Read the model definition and answer for the solid it produces. Units are mm, in the model's axes. A direction names the side the tool comes from. Coordinates: 2 decimals unless noted, no trailing zeros. Write each loop counter-clockwise with the first axis right and the second up, starting at its lowest first coordinate (ties: lowest second). Pieces come first, ordered by that corner, then holes.
(1) Which of the six approach directions +Z, -Z, +X, -X, +Y, -Y give full straight-line access (tool end or side, diameter ignored) to faces 5 (the flat face through (0, 5, 4)), 6 (the flat face through (-0.11, 8.09, -63.03)), 7 (the flat face through (-7.5, 3, -42)), 8 (the flat face through (42, 3, 7.5))?
(2) Given pin 1 (5 mm diameter, centred on x = 34.5, y = 6.5, fed in from -Z); pin 2 (8 mm diameter, centred on x = 3.5, z = -29, fed in from -Y), each flat-ended and moving along its own axis, determine where each tip first touches the part or whether it passes through.
(3) Determine the mould class of faces 1 (the cylindrical face through (-10.568, 2.465, 10.645)), 2 (the flat face through (42, 3, -7.5)), 3 (the flat face through (-7.5, 3, 42)), 4 (the cylindrical face through (63.49, 5.68, -0.09)) for opening direction Z: pulls with the +Z half, pulls with the -Z half, needs draft (parallel to the pull), parting line crosses it, or undercut.
(4) The part is cut by section C-C, the plane z = -49.5. Determine the outline of the cut face in (x, y).
(5) Straight lines are drawn through the part: line 1 along Y through (x, z) = (-7, -33); line 2 along X through (y, z) = (2, -23). For each, find the intervals that lie inside material, in ascending order.
(6) The part is cut by section A-A, the plane z = 0. Determine the outline of the cut face in (x, y).
(7) The part is cut by section B-B, the plane x = 0. Determine the outline of the cut face in (y, z).
(8) The part is cut by section D-D, the plane x = -31.5. Determine the outline of the cut face in (y, z), and give its area (3 significant figures).
```python
from build123d import *

# Parameters (mm, degrees)
EXTRUDE_1_DEPTH             = 5
EXTRUDE_6_DEPTH             = 15
EXTRUDE_7_DEPTH             = 15
EXTRUDE_8_DEPTH             = 15
EXTRUDE_9_DEPTH             = 15
HOLE_WIZARD_M61_D           = 5
HOLE_WIZARD_M51_D           = 4.2
HOLE_WIZARD_M51_ON_FACE_2_D = 4.2
HOLE_WIZARD_M51_ON_FACE_3_D = 4.2
HOLE_WIZARD_M51_ON_FACE_4_D = 4.2


with BuildPart() as part:
    # Эскиз1 → Бобышка-Вытянуть1 (new body)
    with BuildSketch(Plane(origin=(0, 0, 0), x_dir=(1, 0, 0), z_dir=(0, 1, 0))):
        with BuildLine():
            Line((-7.5, 51.5), (7.5, 51.5))
            Line((7.5, 51.5), (7.5, 12.990381057))
            ThreePointArc((7.5, 12.990381057), (10.606601718, 10.606601718), (12.990381057, 7.5))
            Line((12.990381057, 7.5), (51.5, 7.5))
            Line((51.5, 7.5), (51.5, -7.5))
            Line((51.5, -7.5), (12.990381057, -7.5))
            ThreePointArc((12.990381057, -7.5), (10.606601718, -10.606601718), (7.5, -12.990381057))
            Line((7.5, -12.990381057), (7.5, -51.5))
            Line((7.5, -51.5), (-7.5, -51.5))
            Line((-7.5, -51.5), (-7.5, -12.990381057))
            ThreePointArc((-7.5, -12.990381057), (-10.606601718, -10.606601718), (-12.990381057, -7.5))
            Line((-12.990381057, -7.5), (-51.5, -7.5))
            Line((-51.5, -7.5), (-51.5, 7.5))
            Line((-51.5, 7.5), (-12.990381057, 7.5))
            ThreePointArc((-12.990381057, 7.5), (-10.606601718, 10.606601718), (-7.5, 12.990381057))
            Line((-7.5, 12.990381057), (-7.5, 51.5))
        make_face()
    extrude(amount=EXTRUDE_1_DEPTH)

    # Эскиз2 → Бобышка-Вытянуть6 (add)
    with BuildSketch(Plane(origin=(7.5, 0, 0), x_dir=(0, 0, -1), z_dir=(1, 0, 0))):
        Polygon((-51.5, 0), (-71.410254038, 5.334936491), (-70.160254038, 10), (-51.5, 5), align=None)
    extrude(amount=-EXTRUDE_6_DEPTH)

    # Эскиз3 → Бобышка-Вытянуть7 (add)
    with BuildSketch(Plane(origin=(0, 0, -7.5), x_dir=(-1, 0, 0), z_dir=(0, 0, -1))):
        Polygon((-51.5, 0), (-71.410254038, 5.334936491), (-70.160254038, 10), (-51.5, 5), align=None)
    extrude(amount=-EXTRUDE_7_DEPTH)

    # Эскиз4 → Бобышка-Вытянуть8 (add)
    with BuildSketch(Plane.ZY.offset(7.5)):
        Polygon((-51.5, 0), (-71.410254038, 5.334936491), (-70.160254038, 10), (-51.5, 5), align=None)
    extrude(amount=-EXTRUDE_8_DEPTH)

    # Эскиз5 → Бобышка-Вытянуть9 (add)
    with BuildSketch(Plane.XY.offset(7.5)):
        Polygon((-51.5, 0), (-71.410254038, 5.334936491), (-70.160254038, 10), (-51.5, 5), align=None)
    extrude(amount=-EXTRUDE_9_DEPTH)

    # Отверстие обработанное метчиком M61 (through all)
    with Locations(Plane(origin=(0, 5, 0), x_dir=(1, 0, 0), z_dir=(0, 1, 0))):
        with Locations((0, 0)):
            Hole(HOLE_WIZARD_M61_D / 2)

    # Отверстие обработанное метчиком M51 (through all)
    with Locations(Plane(origin=(-60.830127019, 7.5, 0), x_dir=(0.965925826289, -0.258819045103, 0), z_dir=(0.258819045103, 0.965925826289, 0))):
        with Locations((0, 0)):
            Hole(HOLE_WIZARD_M51_D / 2)

    # Отверстие обработанное метчиком M51 on face 2 (through all)
    with Locations(Plane(origin=(0, 7.5, 60.830127019), x_dir=(0, 0.258818959594, 0.965925849201), z_dir=(0, 0.965925849201, -0.258818959594))):
        with Locations((0, 0)):
            Hole(HOLE_WIZARD_M51_ON_FACE_2_D / 2)

    # Отверстие обработанное метчиком M51 on face 3 (through all)
    with Locations(Plane(origin=(60.830127019, 7.5, 0), x_dir=(0.965925849201, 0.258818959594, 0), z_dir=(-0.258818959594, 0.965925849201, 0))):
        with Locations((0, 0)):
            Hole(HOLE_WIZARD_M51_ON_FACE_3_D / 2)

    # Отверстие обработанное метчиком M51 on face 4 (through all)
    with Locations(Plane(origin=(0, 7.5, -60.830127019), x_dir=(0, -0.258818959594, 0.965925849201), z_dir=(0, 0.965925849201, 0.258818959594))):
        with Locations((0, 0)):
            Hole(HOLE_WIZARD_M51_ON_FACE_4_D / 2)


solid = part.part
```
Computed:
1. face 5: +Y
1. face 6: +X, -X, +Y
1. face 7: -Z, -X, +Y, -Y
1. face 8: +Z, +X, +Y, -Y
2. pin 1: stops at z = -7.5
2. pin 2: stops at y = 0
3. face 1: pulls with the +Z half
3. face 2: pulls with the -Z half
3. face 3: needs draft
3. face 4: undercut
4. outline: (-7.5, 0) - (7.5, 0) - (7.5, 5) - (-7.5, 5) - close
5. line 1: y = 0 to 5
5. line 2: x = -7.5 to 7.5
6. outline: (-71.41, 5.33) - (-64.11, 3.38) - (-62.86, 8.04) - (-70.16, 10) - close; (-60.05, 2.29) - (-51.5, 0) - (-2.5, 0) - (-2.5, 5) - (-51.5, 5) - (-58.8, 6.96) - close; (2.5, 0) - (51.5, 0) - (60.05, 2.29) - (58.8, 6.96) - (51.5, 5) - (2.5, 5) - close; (62.86, 8.04) - (64.11, 3.38) - (71.41, 5.33) - (70.16, 10) - close
7. outline: (0, -51.5) - (2.29, -60.05) - (6.96, -58.8) - (5, -51.5) - (5, -2.5) - (0, -2.5) - close; (0, 2.5) - (5, 2.5) - (5, 51.5) - (6.96, 58.8) - (2.29, 60.05) - (0, 51.5) - close; (3.38, -64.11) - (5.33, -71.41) - (10, -70.16) - (8.04, -62.86) - close; (3.38, 64.11) - (8.04, 62.86) - (10, 70.16) - (5.33, 71.41) - close
8. outline: (0, -7.5) - (5, -7.5) - (5, 7.5) - (0, 7.5) - close
8. area: 75.0 mm2
